Part model, mm, in its own coordinate system. A direction names the side the tool comes from. Give positions to 0.01 mm unless a question says otherwise; leave off trailing zeros. Order: outer loops, then holes, each group sorted by start corner. A loop starts at its lowest first (then second) coordinate and runs counter-clockwise, first axis right, second up.
Autodesk Fusion 360 part; units mm, degrees
sketch "Sketch1" plane through (0, 0, 0) normal (0, 0, 1) x (1, 0, 0)
  line L0 (10, 9) -> (-10, 9)
  line L1 (-10, 9) -> (-10, -9)
  line L2 (-10, -9) -> (10, -9)
  line L3 (10, -9) -> (10, 9)
  line L4 (10, 9) -> (-10, -9) construction
  line L5 (-10, 9) -> (10, -9) construction
  line L6 (10, 9) -> (12, 9)
  line L7 (12, 9) -> (12, -9)
  line L8 (12, -9) -> (10, -9)
  line L9 (10, -9) -> (10, 9)
  line L10 (-10, 9) -> (-12, 9)
  line L11 (-12, 9) -> (-12, -9)
  line L12 (-12, -9) -> (-10, -9)
  line L13 (-10, -9) -> (-10, 9)
  dimension "d1" = 20
  dimension "d2" = 18
  dimension "d3" = 2
extrude "Extrude1" add sketch "Sketch1" along normal blind 2 contours L0 L1 L2 L3 L9 L13
extrude "Extrude2" add sketch "Sketch1" along normal blind 22.6 contours L3 L6 L7 L8 L9 | L1 L10 L11 L12 L13
sketch "Sketch2" plane through (0, -9, 0) normal (0, -1, 0) x (1, 0, 0)
  line L0 (-12, 0) -> (12, 0)
  line L1 (12, 0) -> (12, 22.6)
  line L2 (12, 22.6) -> (10, 22.6)
  line L3 (10, 22.6) -> (10, 2)
  line L4 (10, 2) -> (-10, 2)
  line L5 (-10, 2) -> (-10, 22.6)
  line L6 (-10, 22.6) -> (-12, 22.6)
  line L7 (-12, 22.6) -> (-12, 0)
  line L8 (-12, 22.6) -> (-8, 22.6)
  line L9 (-8, 22.6) -> (-8, 24.6)
  line L10 (-8, 24.6) -> (-12, 24.6)
  line L11 (-12, 24.6) -> (-12, 22.6)
  line L12 (12, 22.6) -> (8, 22.6)
  line L13 (8, 22.6) -> (8, 24.6)
  line L14 (8, 24.6) -> (12, 24.6)
  line L15 (12, 24.6) -> (12, 22.6)
  dimension "d8" = 4
  dimension "d9" = 2
  dimension "d10" = 4
  dimension "d11" = 2
extrude "Extrude3" add sketch "Sketch2" against normal blind 18 contours L6 L8 L9 L10 L11 | L2 L12 L13 L14 L15
Item 1: Pull direction Z, two halves, no side cores. Call faces 1 (the face through (-10, 0, 12)), 2 (the face through (10, 0, 24.6)), 3 (the face through (9, 0, 22.6)), 4 (the face through (8, 0, 24)): released by +Z, released by -Z, zero draft, split by the parting line, or undercut.
Item 2: Drill centre lines: probe 1 along X at (y, z) = (-7.25, 12.75); probe 2 along Z at (x, y) = (-9.75, 5.25); probe 3 along Z at (x, y) = (2.5, -3.75). Where is each one in solid material? Low to high.
Item 3: Which spindle directions (+Z, -Z, +X, -X, +Y, -Y) get a long thin tool onto all of the face, cutting with end or side? Do faces 5 (the face through (0, 0, 0)), 6 (the face through (0, 0, 2)), 7 (the face through (-8, 0, 24)). Say none if no direction does.
Item 4: Band-saw the part on A-A on z = 22.25. List the corners of the cut face in (x, y), plus the area to 3 significant figures.
Item 5: Band-saw the part on B-B on y = -6.25. List the corners of the cut face in (x, z), plus the area to 3 significant figures.
Item 6: Band-saw the part on C-C on x = 4. List the corners of the cut face in (y, z).
Item 7: Drop a flat-ended pin along its axis: P1, Ø6, axis at x = 2.5, y = 1, coming from the +Z side. Give the stop position or say it passes through.
Working result:
1. face 1: undercut
1. face 2: released by +Z
1. face 3: undercut
1. face 4: zero draft
2. probe 1: x = -12 to -10, 10 to 12
2. probe 2: z = 0 to 2, 22.6 to 24.6
2. probe 3: z = 0 to 2
3. face 5: -Z, +X, -X, +Y, -Y
3. face 6: +Y, -Y
3. face 7: +Z, +Y, -Y
4. outline: (-12, -9) - (-10, -9) - (-10, 9) - (-12, 9) - close; (10, -9) - (12, -9) - (12, 9) - (10, 9) - close
4. area: 72.0 mm2
5. outline: (-12, 0) - (12, 0) - (12, 24.6) - (8, 24.6) - (8, 22.6) - (10, 22.6) - (10, 2) - (-10, 2) - (-10, 22.6) - (-8, 22.6) - (-8, 24.6) - (-12, 24.6) - close
5. area: 146 mm2
6. outline: (-9, 0) - (9, 0) - (9, 2) - (-9, 2) - close
7. P1: stops at z = 2
